```python
from build123d import *

# Parameters (mm, degrees)
BOSS_EXTRUDE1_DEPTH            = 30
SKETCH2_R                      = 2.6
SKETCH2_R_2                    = 1.55
BOSS_EXTRUDE3_DEPTH            = 5
CUT_EXTRUDE1_REACH             = 108.419
CUT_EXTRUDE1_DIRECTION_2_DEPTH = 107.419489108
CUT_EXTRUDE2_REACH             = 108.419
CUT_EXTRUDE2_DIRECTION_2_DEPTH = 107.419489108
FILLET1_R                      = 2
SKETCH6_R                      = 1.55
BOSS_EXTRUDE4_DEPTH            = 1


with BuildPart() as part:
    # Sketch1 → Boss-Extrude1 (new body)
    with BuildSketch(Plane(origin=(0, 0, 0), x_dir=(1, 0, 0), z_dir=(0, 1, 0))):
        Polygon((-13.5, 0), (0, 92.188031325), (13.5, 0), (14.489447114, 0.144894471), (0, 99.089605913), (-14.489447114, 0.144894471), align=None)
    extrude(amount=BOSS_EXTRUDE1_DEPTH)

    # Sketch2 → Boss-Extrude3 (add)
    # profile 1 of 10: a face of its own
    with BuildSketch(Plane(origin=(0, 0, 0), x_dir=(1, 0, 0), z_dir=(0, 1, 0))):
        with Locations((11.916884617, -0.231831154)):
            Circle(SKETCH2_R)
        with Locations(Location((11.916884617, -0.231831154, 0), (0, 0, 270))):
            Circle(SKETCH2_R_2, mode=Mode.SUBTRACT)
    # profile 2 of 10: a face of its own
    with BuildSketch(Plane(origin=(0, 0, 0), x_dir=(1, 0, 0), z_dir=(0, 1, 0))):
        with Locations((9.888362021, 13.620428448)):
            Circle(SKETCH2_R)
        with Locations(Location((9.888362021, 13.620428448, 0), (0, 0, 270))):
            Circle(SKETCH2_R_2, mode=Mode.SUBTRACT)
    # profile 3 of 10: a face of its own
    with BuildSketch(Plane(origin=(0, 0, 0), x_dir=(1, 0, 0), z_dir=(0, 1, 0))):
        with Locations((7.859839425, 27.47268805)):
            Circle(SKETCH2_R)
        with Locations(Location((7.859839425, 27.47268805, 0), (0, 0, 270))):
            Circle(SKETCH2_R_2, mode=Mode.SUBTRACT)
    # profile 4 of 10: a face of its own
    with BuildSketch(Plane(origin=(0, 0, 0), x_dir=(1, 0, 0), z_dir=(0, 1, 0))):
        with Locations((5.831316829, 41.324947652)):
            Circle(SKETCH2_R)
        with Locations(Location((5.831316829, 41.324947652, 0), (0, 0, 270))):
            Circle(SKETCH2_R_2, mode=Mode.SUBTRACT)
    # profile 5 of 10: a face of its own
    with BuildSketch(Plane(origin=(0, 0, 0), x_dir=(1, 0, 0), z_dir=(0, 1, 0))):
        with Locations((3.802794233, 55.177207254)):
            Circle(SKETCH2_R)
        with Locations(Location((3.802794233, 55.177207254, 0), (0, 0, 270))):
            Circle(SKETCH2_R_2, mode=Mode.SUBTRACT)
    # profile 6 of 10: a face of its own
    with BuildSketch(Plane(origin=(0, 0, 0), x_dir=(1, 0, 0), z_dir=(0, 1, 0))):
        with Locations((-11.916884617, -0.231831154)):
            Circle(SKETCH2_R)
        with Locations(Location((-11.916884617, -0.231831154, 0), (0, 0, 90))):
            Circle(SKETCH2_R_2, mode=Mode.SUBTRACT)
    # profile 7 of 10: a face of its own
    with BuildSketch(Plane(origin=(0, 0, 0), x_dir=(1, 0, 0), z_dir=(0, 1, 0))):
        with Locations((-9.888362021, 13.620428448)):
            Circle(SKETCH2_R)
        with Locations(Location((-9.888362021, 13.620428448, 0), (0, 0, 90))):
            Circle(SKETCH2_R_2, mode=Mode.SUBTRACT)
    # profile 8 of 10: a face of its own
    with BuildSketch(Plane(origin=(0, 0, 0), x_dir=(1, 0, 0), z_dir=(0, 1, 0))):
        with Locations((-7.859839425, 27.47268805)):
            Circle(SKETCH2_R)
        with Locations(Location((-7.859839425, 27.47268805, 0), (0, 0, 90))):
            Circle(SKETCH2_R_2, mode=Mode.SUBTRACT)
    # profile 9 of 10: a face of its own
    with BuildSketch(Plane(origin=(0, 0, 0), x_dir=(1, 0, 0), z_dir=(0, 1, 0))):
        with Locations((-5.831316829, 41.324947652)):
            Circle(SKETCH2_R)
        with Locations(Location((-5.831316829, 41.324947652, 0), (0, 0, 90))):
            Circle(SKETCH2_R_2, mode=Mode.SUBTRACT)
    # profile 10 of 10: a face of its own
    with BuildSketch(Plane(origin=(0, 0, 0), x_dir=(1, 0, 0), z_dir=(0, 1, 0))):
        with Locations((-3.802794233, 55.177207254)):
            Circle(SKETCH2_R)
        with Locations(Location((-3.802794233, 55.177207254, 0), (0, 0, 90))):
            Circle(SKETCH2_R_2, mode=Mode.SUBTRACT)
    boss_extrude3 = extrude(amount=BOSS_EXTRUDE3_DEPTH)

    # Cut-Extrude1: up to this face of the body (flat: up to its plane)
    cut_extrude1_end = Plane(part.part.faces().sort_by_distance((-6.674060715, 15.426495801, -46.612585527))[0])
    # Sketch4 → Cut-Extrude1 (cut, up to the picked face)
    with BuildSketch(Plane(origin=(0.283424505, 0, 1.935433121), x_dir=(0.9894471144188783, 0, -0.14489447114419254), z_dir=(0.14489447114419252, 0, 0.9894471144188782)), mode=Mode.PRIVATE) as cut_extrude1_sk1:
        Polygon((13.357536045, 5), (9.157536045, 5), (9.157536045, 1.475781549), align=None)
    cut_extrude1_tool1 = split(extrude(cut_extrude1_sk1.sketch, amount=-CUT_EXTRUDE1_REACH, mode=Mode.PRIVATE), bisect_by=cut_extrude1_end, keep=Keep.BOTH, mode=Mode.PRIVATE)
    cut_extrude1 = cut_extrude1_tool1.solids().sort_by(Axis((10.729548, 3.825261, 0.405705), (-0.14489447114419252, 0, -0.9894471144188782)))[0]
    add(cut_extrude1, mode=Mode.SUBTRACT)

    # Sketch4 → Cut-Extrude1 direction 2 (cut)
    with BuildSketch(Plane(origin=(0.283424505, 0, 1.935433121), x_dir=(0.9894471144188783, 0, -0.14489447114419254), z_dir=(0.14489447114419252, 0, 0.9894471144188782))):
        Polygon((13.357536045, 5), (9.157536045, 5), (9.157536045, 1.475781549), align=None)
    cut_extrude1_direction_2 = extrude(amount=CUT_EXTRUDE1_DIRECTION_2_DEPTH, mode=Mode.SUBTRACT)

    # Cut-Extrude2: up to this face of the body (flat: up to its plane)
    cut_extrude2_end = Plane(part.part.faces().sort_by_distance((6.674060715, 15.426495801, -46.612585527))[0])
    # Sketch5 → Cut-Extrude2 (cut, up to the picked face)
    with BuildSketch(Plane(origin=(-0.283424505, 0, 1.935433121), x_dir=(0.9894471144188784, 0, 0.14489447114419146), z_dir=(-0.14489447114419146, 0, 0.9894471144188784)), mode=Mode.PRIVATE) as cut_extrude2_sk1:
        Polygon((-9.157536045, 5), (-9.157536045, 1.475781549), (-13.357536045, 5), align=None)
    cut_extrude2_tool1 = split(extrude(cut_extrude2_sk1.sketch, amount=-CUT_EXTRUDE2_REACH, mode=Mode.PRIVATE), bisect_by=cut_extrude2_end, keep=Keep.BOTH, mode=Mode.PRIVATE)
    cut_extrude2 = cut_extrude2_tool1.solids().sort_by(Axis((-10.729548, 3.825261, 0.405705), (0.14489447114419146, 0, -0.9894471144188784)))[0]
    add(cut_extrude2, mode=Mode.SUBTRACT)

    # Sketch5 → Cut-Extrude2 direction 2 (cut)
    with BuildSketch(Plane(origin=(-0.283424505, 0, 1.935433121), x_dir=(0.9894471144188784, 0, 0.14489447114419146), z_dir=(-0.14489447114419146, 0, 0.9894471144188784))):
        Polygon((-9.157536045, 5), (-9.157536045, 1.475781549), (-13.357536045, 5), align=None)
    cut_extrude2_direction_2 = extrude(amount=CUT_EXTRUDE2_DIRECTION_2_DEPTH, mode=Mode.SUBTRACT)

    # Mirror2: Boss-Extrude3, Cut-Extrude1, Cut-Extrude1 direction 2, Cut-Extrude2, Cut-Extrude2 direction 2 across plane
    add(boss_extrude3.mirror(Plane.ZX.offset(15)))
    add(cut_extrude1.mirror(Plane.ZX.offset(15)), mode=Mode.SUBTRACT)
    add(cut_extrude1_direction_2.mirror(Plane.ZX.offset(15)), mode=Mode.SUBTRACT)
    add(cut_extrude2.mirror(Plane.ZX.offset(15)), mode=Mode.SUBTRACT)
    add(cut_extrude2_direction_2.mirror(Plane.ZX.offset(15)), mode=Mode.SUBTRACT)

    # Fillet1
    # the kernel refuses this fillet: 2 mm, written as the material it adds along each edge
    with BuildSketch(Plane(origin=(13.5, 5, 0), x_dir=(0, 1, 0), z_dir=(0.9894471144188783, 0, -0.1448944711441925))) as fillet1_piece_1_section:
        with BuildLine():
            CenterArc((FILLET1_R, FILLET1_R), FILLET1_R, 180, 90)
            Line((0, FILLET1_R), (0, 0))
            Line((0, 0), (FILLET1_R, 0))
        make_face()
    fillet1_piece_1 = extrude(amount=6, mode=Mode.PRIVATE)
    fillet1_piece_1 = fillet1_piece_1 & Plane(origin=(11.916884617, 5.699977741, 0.231831154), x_dir=(1, 0, 0), z_dir=(0, -1, 0)) * Cylinder(2.6, 20, mode=Mode.PRIVATE)
    add(fillet1_piece_1)
    with BuildSketch(Plane(origin=(13.5, 25, 0), x_dir=(0, -1, 0), z_dir=(0.9894471144188783, 0, -0.1448944711441925))) as fillet1_piece_2_section:
        with BuildLine():
            CenterArc((FILLET1_R, -FILLET1_R), FILLET1_R, 90, 90)
            Line((0, -FILLET1_R), (0, 0))
            Line((0, 0), (FILLET1_R, 0))
        make_face()
    fillet1_piece_2 = extrude(amount=6, mode=Mode.PRIVATE)
    fillet1_piece_2 = fillet1_piece_2 & Plane(origin=(11.916884617, 24.30002226, 0.231831154), x_dir=(1, 0, 0), z_dir=(0, 1, 0)) * Cylinder(2.6, 20, mode=Mode.PRIVATE)
    add(fillet1_piece_2)
    with BuildSketch(Plane(origin=(-19.436682687, 25, -0.869366827), x_dir=(0, -1, 0), z_dir=(0.9894471144188784, 0, 0.1448944711441914))) as fillet1_piece_3_section:
        with BuildLine():
            CenterArc((FILLET1_R, -FILLET1_R), FILLET1_R, 90, 90)
            Line((0, -FILLET1_R), (0, 0))
            Line((0, 0), (FILLET1_R, 0))
        make_face()
    fillet1_piece_3 = extrude(amount=6, mode=Mode.PRIVATE)
    fillet1_piece_3 = fillet1_piece_3 & Plane(origin=(-11.916884617, 24.777637105, 0.231831154), x_dir=(1, 0, 0), z_dir=(0, 1, 0)) * Cylinder(2.6, 21, mode=Mode.PRIVATE)
    add(fillet1_piece_3)
    with BuildSketch(Plane(origin=(-19.436682687, 5, -0.869366827), x_dir=(-0.1448944711441914, 0, 0.9894471144188784), z_dir=(0.9894471144188784, 0, 0.1448944711441914))) as fillet1_piece_4_section:
        with BuildLine():
            CenterArc((FILLET1_R, -FILLET1_R), FILLET1_R, 90, 90)
            Line((0, -FILLET1_R), (0, 0))
            Line((0, 0), (FILLET1_R, 0))
        make_face()
    fillet1_piece_4 = extrude(amount=6, mode=Mode.PRIVATE)
    fillet1_piece_4 = fillet1_piece_4 & Plane(origin=(-11.916884617, 5.222362792, 0.231831154), x_dir=(1, 0, 0), z_dir=(0, -1, 0)) * Cylinder(2.6, 21, mode=Mode.PRIVATE)
    add(fillet1_piece_4)

    # Sketch6 → Boss-Extrude4 (add)
    with BuildSketch(Plane.XZ):
        with Locations(Location((3.802794233, -55.177207254, 0), (0, 0, 270))):
            Circle(SKETCH6_R)
        with Locations(Location((-3.802794233, -55.177207254, 0), (0, 0, 270))):
            Circle(SKETCH6_R)
        with Locations(Location((-5.831316829, -41.324947652, 0), (0, 0, 270))):
            Circle(SKETCH6_R)
        with Locations(Location((5.831316829, -41.324947652, 0), (0, 0, 270))):
            Circle(SKETCH6_R)
        with Locations(Location((7.859839425, -27.47268805, 0), (0, 0, 270))):
            Circle(SKETCH6_R)
        with Locations(Location((-7.859839425, -27.47268805, 0), (0, 0, 270))):
            Circle(SKETCH6_R)
        with Locations(Location((-9.888362021, -13.620428448, 0), (0, 0, 270))):
            Circle(SKETCH6_R)
        with Locations(Location((9.888362021, -13.620428448, 0), (0, 0, 270))):
            Circle(SKETCH6_R)
        with Locations(Location((11.916884617, 0.231831154, 0), (0, 0, 270))):
            Circle(SKETCH6_R)
        with Locations(Location((-11.916884617, 0.231831154, 0), (0, 0, 270))):
            Circle(SKETCH6_R)
    extrude(amount=-BOSS_EXTRUDE4_DEPTH)


solid = part.part
```
Work out the finished part from the listing and answer in its coordinate system (mm). A direction names the side the tool comes from. Give positions to 0.01 mm unless a question says otherwise; leave off trailing zeros. Order: outer loops, then holes, each group sorted by start corner. A loop starts at its lowest first (then second) coordinate and runs counter-clockwise, first axis right, second up. Notation, with made-up numbers: (30, 61) -> (63, 61) arc R29 ccw to (63, 89) -> close; hole circle Ø7 at (-16, 15.5). An arc over 180 degrees is marked (long way). Answer as CSV lines item,"result". Start each with the question number.
(1) For a pull along Z with two mould halves and no side action, classify faces 1 (the cylindrical face through (-1.77, 28.646, -53.556)), 2 (the flat face through (7.346, 14.79, -48.925)), 3 (the flat face through (-4.22, 2.43, -42.22)) as released by +Z, released by -Z, zero draft, split by the parting line, or undercut.
(2) Consider line 1 along Y through (x, z) = (7.75, -12.5); line 2 along X through (y, z) = (25.5, -55); line 3 along X through (y, z) = (17, -77.5). Determine where each line is inside the solid, lowest interval first.
(3) Section C-C, the plane y = 24 is taken. Write down the section's boundary in (x, z).
(4) Which of the six approach directions +Z, -Z, +X, -X, +Y, -Y give full straight-line access (tool end or side, diameter ignored) to faces 4 (the flat face through (4.22, 2.43, -42.22)), 5 (the cylindrical face through (-13.946, 5.835, 0.313)), 6 (the flat face through (-12, 1, 0)), 7 (the cylindrical face through (14.042, 5.835, 0.299))?
(5) Section A-A, the plane z = -9 is taken. Write down the section's boundary in (x, y), plus the area to 3 significant figures.
(6) Section B-B, the plane y = 18.5 is taken. Write down the section's boundary in (x, z), plus the area to 3 significant figures.
(7) Each of these flat-tipped pins is pushed along its axis until it touches: pin 1 Ø2.5 at (x, z) = (-10.5, -13.5) entering from +Y; pin 2 Ø0.9 at (x, z) = (12, 1) entering from +Y; pin 3 Ø5 at (y, z) = (22.5, -39.5) entering from -X; pin 4 Ø1.5 at (y, z) = (23, -77.5) entering from +X. Where does it stop, or does it pass through?
Entries:
1,face 1,"undercut"
1,face 2,"released by -Z"
1,face 3,"released by +Z"
2,line 1,"0 to 1.75, 28.25 to 30"
2,line 2,"-6.46 to -5.34, 5.34 to 6.46"
2,line 3,"-3.16 to -2.15, 2.15 to 3.16"
3,outline,"(-14.51, 0.12) arc R2.6 ccw to (-14.49, -0.14) -> (0, -99.09) -> (14.49, -0.14) arc R2.6 ccw to (14.51, 0.12) -> (13.54, 0.27) -> (0, -92.19) -> (-13.54, 0.27) -> close"
4,face 4,"+Z"
4,face 5,"+Z, -X"
4,face 6,"+Y"
4,face 7,"+Z, +X"
5,outline,"(-13.19, 0) -> (-12.18, 0) -> (-12.18, 30) -> (-13.19, 30) -> close; (12.18, 0) -> (13.19, 0) -> (13.19, 30) -> (12.18, 30) -> close"
5,area,"60.6 mm²"
6,outline,"(-14.49, -0.14) -> (0, -99.09) -> (14.49, -0.14) -> (13.5, 0) -> (0, -92.19) -> (-13.5, 0) -> close"
6,area,"193 mm²"
7,pin 1,"y = 30"
7,pin 2,"y = 1"
7,pin 3,"x = -9.09"
7,pin 4,"x = 3.27"
